Build history of the part. All positions in model axes, mm. Face numbers are marked on the shaded views. A direction names the side the tool comes from. Round coordinates to 2 decimals unless told otherwise and drop trailing zeros. Loops run counter-clockwise (first coordinate to the right, second up) from the corner with the lowest first, then second, coordinate; pieces in that order, holes last. Notation, with made-up numbers: (-23.5, 41) -> (3.5, 41) arc R27 ccw to (3.5, 78) -> close; hole circle Ø10 at (88, 32). An arc over 180 degrees is marked (long way). Put each result on its own line as item: value. Start each with the question number.
```python
from build123d import *

# Parameters (mm, degrees)
F4_DEPTH = 10.16


with BuildPart() as f1:
    # F0 (on Front) → F1 (revolve)
    with BuildSketch(Plane.XZ):
        with BuildLine():
            Line((25.781, 19.05), (25.781, 0))
            Line((25.781, 0), (31.4325, 0))
            Line((31.4325, 0), (31.4325, 4.826))
            Line((31.4325, 4.826), (40.005, 4.826))
            Line((40.005, 4.826), (40.005, 12.7))
            ThreePointArc((40.005, 12.7), (38.1451280605, 17.1901280605), (33.655, 19.05))
            Line((33.655, 19.05), (25.781, 19.05))
        make_face()
    revolve(axis=Axis((0, 0, 5.4042546308), (0, 0, -1)))

    # F3 (on offset) → F4 (cut)
    with BuildSketch(Plane.XY.offset(19.05)):
        with BuildLine():
            ThreePointArc((9.084087807, 38.9599714286), (0, 40.005), (-9.084087807, 38.9599714286))
            ThreePointArc((-9.084087807, 38.9599714286), (0, 30.861), (9.084087807, 38.9599714286))
        make_face()
        with BuildLine():
            ThreePointArc((-36.1239683258, 17.1889190294), (-24.1281013804, 19.2415187752), (-24.7962961121, 31.3933707034))
            ThreePointArc((-24.7962961121, 31.3933707034), (-31.2771684561, 24.9427095234), (-36.1239683258, 17.1889190294))
        make_face()
        with BuildLine():
            ThreePointArc((-35.9617639006, -17.5257399889), (-30.0872502978, -6.8672185428), (-40.0045633065, 0.1869215305))
            ThreePointArc((-40.0045633065, 0.1869215305), (-39.0019911268, -8.9019499629), (-35.9617639006, -17.5257399889))
        make_face()
        with BuildLine():
            ThreePointArc((-8.719617772, -39.0431593357), (-13.3900860729, -27.8048002323), (-25.0885783867, -31.1602833673))
            ThreePointArc((-25.0885783867, -31.1602833673), (-17.3575189834, -36.0432595604), (-8.719617772, -39.0431593357))
        make_face()
        with BuildLine():
            ThreePointArc((25.0885783867, -31.1602833673), (13.3900860729, -27.8048002323), (8.719617772, -39.0431593357))
            ThreePointArc((8.719617772, -39.0431593357), (17.3575189834, -36.0432595604), (25.0885783867, -31.1602833673))
        make_face()
        with BuildLine():
            ThreePointArc((40.0045633065, 0.1869215305), (30.0872502978, -6.8672185428), (35.9617639006, -17.5257399889))
            ThreePointArc((35.9617639006, -17.5257399889), (39.0019911268, -8.9019499629), (40.0045633065, 0.1869215305))
        make_face()
        with BuildLine():
            ThreePointArc((24.7962961121, 31.3933707034), (24.1281013804, 19.2415187752), (36.1239683258, 17.1889190294))
            ThreePointArc((36.1239683258, 17.1889190294), (31.2771684561, 24.9427095234), (24.7962961121, 31.3933707034))
        make_face()
    extrude(amount=-F4_DEPTH, mode=Mode.SUBTRACT)


solid = f1.part
```
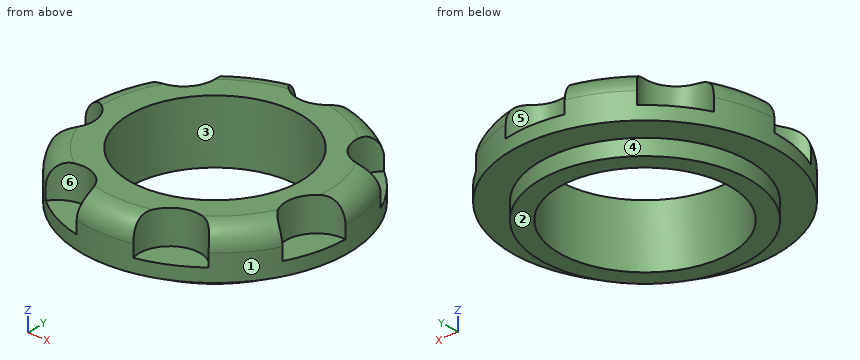
Item 1: Cut at B-B on z = 1.5. Write the cut outline in (x, y) (1 decimal).
Item 2: Wall check: line 1 (X direction, y = 0, z = 8) (3 decimals); line 2 (Y direction, x = -6, z = 16.25); line 3 (Y direction, x = -6, z = 6). Give the ranges that are in metal, low to high. Write a range as from..to.
Item 3: Drop flat-ended pins along their axis: pin 1 (7 mm diameter, centred on x = -26.5, y = 23.5, fed in from +Z); pin 2 (2 mm diameter, centred on x = -30.5, y = -19, fed in from -Z); pin 3 (4 mm diameter, centred on y = -12.5, z = 6.5, fed in from +X). Give the stop position or say it passes through.
Item 4: Cut at C-C on z = 10.5. Write the cut outline in (x, y) (3 decimals), then the cut area to 4 significant figures.
Item 5: Pull direction Y, two halves, no side cores. Call the marked faces 1, 2 and 3: +Y half, -Y half, draft (parallel to the pull), parting line (faces both ways), or undercut.
Item 6: 3-axis set-ups, long thin cutter, end or side, ignore diameter. For the marked faces 4, 5 and 6: which of +Z, -Z, +X, -X, +Y, -Y reach the whole face in a straight line?
Ans:
1. outline: circle Ø62.9 at (0, 0); hole circle Ø51.6 at (0, 0)
2. line 1: x = -40.005..-25.781, 25.781..40.005
2. line 2: y = -38.45..-25.07, 25.07..33.1
2. line 3: y = -39.55..-25.07, 25.07..39.55
3. pin 1: stops at z = 8.89
3. pin 2: stops at z = 4.83
3. pin 3: stops at x = 38.6
4. outline: (-40.005, 0.187) arc R9.144 cw to (-35.962, -17.526) arc R40.005 ccw to (-25.089, -31.16) arc R9.144 cw to (-8.72, -39.043) arc R40.005 ccw to (8.72, -39.043) arc R9.144 cw to (25.089, -31.16) arc R40.005 ccw to (35.962, -17.526) arc R9.144 cw to (40.005, 0.187) arc R40.005 ccw to (36.124, 17.189) arc R9.144 cw to (24.796, 31.393) arc R40.005 ccw to (9.084, 38.96) arc R9.144 cw to (-9.084, 38.96) arc R40.005 ccw to (-24.796, 31.393) arc R9.144 cw to (-36.124, 17.189) arc R40.005 ccw to start; hole circle Ø51.562 at (0, 0)
4. area: 2,065 mm2
5. face 1: parting line
5. face 2: draft
5. face 3: undercut
6. face 4: -Z
6. face 5: +Z, +Y
6. face 6: +Z
